from build123d import *

# Parameters (mm, degrees)
SKETCH1_R           = 1.7
BOSS_EXTRUDE1_DEPTH = 3


with BuildPart() as part:
    # Sketch1 → Boss-Extrude1 (new body)
    with BuildSketch(Plane.XZ):
        with BuildLine():
            Line((0, 52.5), (0, 48.2))
            ThreePointArc((0, 48.2), (-1.7, 46.5), (0, 44.8))
            Line((0, 44.8), (0, 39.816447761))
            ThreePointArc((0, 39.816447761), (-39.816447761, 0), (0, -39.816447761))
            Line((0, -39.816447761), (0, -44.8))
            ThreePointArc((0, -44.8), (-1.7, -46.5), (0, -48.2))
            Line((0, -48.2), (0, -52.5))
            ThreePointArc((0, -52.5), (-52.5, 0), (0, 52.5))
        make_face()
        with Locations(Location((-46.5, 0, 0), (0, 0, 270))):
            Circle(SKETCH1_R, mode=Mode.SUBTRACT)
        with Locations(Location((-32.880465325, 32.880465325, 0), (0, 0, 270))):
            Circle(SKETCH1_R, mode=Mode.SUBTRACT)
        with Locations(Location((-32.880465325, -32.880465325, 0), (0, 0, 90))):
            Circle(SKETCH1_R, mode=Mode.SUBTRACT)
    extrude(amount=BOSS_EXTRUDE1_DEPTH)


solid = part.part
Read the model definition and answer for the solid it produces. Units are mm, in the model's axes. Round coordinates to 2 decimals unless told otherwise and drop trailing zeros. Order: outer loops, then holes, each group sorted by start corner. A loop starts at its lowest first (then second) coordinate and runs counter-clockwise, first axis right, second up. Notation, with made-up numbers: (26, -38.75) - (59, -38.75) arc R25 ccw to (59, -14.75) - close; hole circle Ø10 at (46, 28.25). An arc over 180 degrees is marked (long way). Use one line per item in the form item = value. Start each with the question number.
(1) Determine the mould class of faces 1 (the face through (0, -1, 42)), 2 (the face through (-32.23, -1.48, -31.31)), 3 (the face through (-40, 0, 4)) for opening direction X: +X half, -X half, draft (parallel to the pull), parting line (faces both ways), or undercut.
(2) The part is cut by section B-B (x = -14). Give the vertices of the cut face in (y, z), then the cut area to 3 significant figures.
(3) A flat-ended cylindrical pin translates along its axis: pin 1 Ø1 at (y, z) = (-0.5, 32) entering from -X. Find the tip coordinate at first contact, or state that the pin passes through.
(4) The part is cut by section C-C (y = -2.35). Give the vertices of the cut face in (x, z).
(5) The part is cut by section D-D (z = -12). Give the vertices of the cut face in (x, y), then the cut area to 3 significant figures.
(6) The part is cut by section A-A (z = 0). Give the vertices of the cut face in (x, y), then the cut area to 3 significant figures.
(7) Find the intervals of material crossed by line 1 along Z through (x, y) = (-32, -1.4); line 2 along X through (y, z) = (-1.05, 0); line 3 along Z through (x, y) = (-33.5, -0.9), in increasing order. Write a range as from..to.
Checked values:
q1.face_1 = +X half
q1.face_2 = undercut
q1.face_3 = draft
q2.outline = (-3, -50.6) - (0, -50.6) - (0, -37.27) - (-3, -37.27) - close; (-3, 37.27) - (0, 37.27) - (0, 50.6) - (-3, 50.6) - close
q2.area = 79.9 mm^2
q3.pin_1 = -42
q4.outline = (0, -52.5) - (0, -48.2) arc R1.7 cw to (0, -44.8) - (0, -39.82) arc R39.82 cw to (0, 39.82) - (0, 44.8) arc R1.7 cw to (0, 48.2) - (0, 52.5) arc R52.5 ccw to start; hole circle Ø3.4 at (-46.5, 0); hole circle Ø3.4 at (-32.88, -32.88); hole circle Ø3.4 at (-32.88, 32.88)
q5.outline = (-51.11, -3) - (-37.97, -3) - (-37.97, 0) - (-51.11, 0) - close
q5.area = 39.4 mm^2
q6.outline = (-52.5, -3) - (-48.2, -3) - (-48.2, 0) - (-52.5, 0) - close; (-44.8, -3) - (-39.82, -3) - (-39.82, 0) - (-44.8, 0) - close
q6.area = 27.9 mm^2
q7.line_1 = -41.62..-34.33, -31.43..-23.69, 23.69..31.43, 34.33..41.62
q7.line_2 = -52.5..-48.2, -44.8..-39.82
q7.line_3 = -40.42..-34.46, -31.3..-21.52, 21.52..31.3, 34.46..40.42
